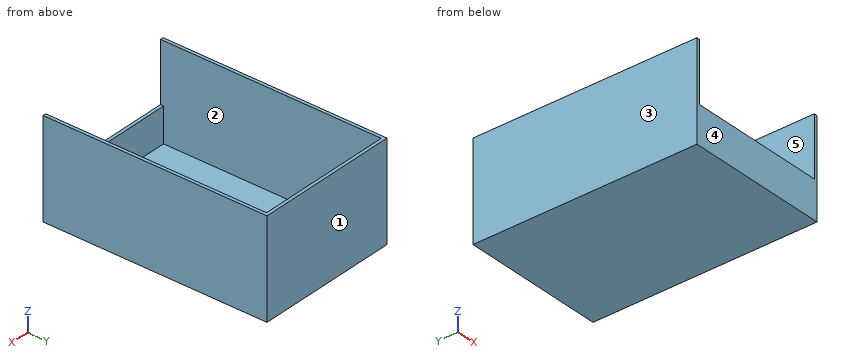
```python
from build123d import *

# Parameters (mm, degrees)
F0_W     = 50.8
F0_H     = 6.35
F0_W_2   = 177.8
F1_DEPTH = 453.39
F2_DEPTH = 6.35
F3_W     = 292.1
F3_H     = 196.85
F4_DEPTH = 6.35


with BuildPart() as f1:
    # F0 (on Front) → F1 (new body)
    with BuildSketch(Plane.XZ):
        Polygon((-139.7, -92.075), (-139.7, -22.225), (-139.7, 98.425), (-146.05, 98.425), (-146.05, -98.425), (-139.7, -98.425), align=None)
        with Locations((-114.3, -95.25)):
            Rectangle(F0_W, F0_H)
        with Locations((114.3, -95.25)):
            Rectangle(F0_W, F0_H)
        Polygon((146.05, -98.425), (146.05, 98.425), (139.7, 98.425), (139.7, -22.225), (139.7, -92.075), (139.7, -98.425), align=None)
        with Locations((0, -95.25)):
            Rectangle(F0_W_2, F0_H)
    extrude(amount=-F1_DEPTH)

    # F0 (on Front) → F2 (join)
    with BuildSketch(Plane.XZ):
        Polygon((139.7, -92.075), (139.7, -22.225), (-139.7, -22.225), (-139.7, -92.075), (-88.9, -92.075), (88.9, -92.075), align=None)
        with Locations((0, -95.25)):
            Rectangle(F0_W_2, F0_H)
        with Locations((-114.3, -95.25)):
            Rectangle(F0_W, F0_H)
        with Locations((114.3, -95.25)):
            Rectangle(F0_W, F0_H)
    extrude(amount=-F2_DEPTH)

    # F3 (on face) → F4 (join)
    with BuildSketch(Plane(origin=(0, 453.39, 0), x_dir=(-1, 0, 0), z_dir=(0, 1, 0))):
        Rectangle(F3_W, F3_H)
    extrude(amount=-F4_DEPTH)


solid = f1.part
```
Geometry check sheet. Reference: the model listing, model coordinates, mm. Face numbers are marked on the shaded views. A direction names the side the tool comes from. Give positions to 0.01 mm unless a question says otherwise; leave off trailing zeros. Order: outer loops, then holes, each group sorted by start corner. A loop starts at its lowest first (then second) coordinate and runs counter-clockwise, first axis right, second up. Notation, with made-up numbers: (31, 72) - (50, 72) arc R33 ccw to (50, 107) - close; hole circle Ø10 at (29.25, 35.5). An arc over 180 degrees is marked (long way). Answer in a Markdown table with one row per item. Add a question column.
Q1. Cross-section at B-B, the plane y = 181.5. Enter the section's corners in (x, z) (3 decimals).
Q2. Cross-section at A-A, the plane z = -76. Enter the section's corners in (x, y), then the cut area to 3 significant figures.
Q3. Tool access check on the marked faces 1 and 2. Record the directions out of +Z, -Z, +X, -X, +Y, -Y that give a thin tool (end or side, any length) a straight path to the whole face; none if there is none.
Q4. Cross-section at C-C, the plane x = 36. Enter the section's corners in (y, z) (3 decimals), then the cut area to 3 significant figures.
Q5. Material ranges on probe 1 along X at (y, z) = (343, -78.5); probe 2 along Y at (x, z) = (-125, -40); probe 3 along Z at (x, y) = (-118, 33.5) (3 decimals), recorded low to high. Write a range as from..to.
Q6. Gauge pin test, flat ends, axial feed: pin 1 (2 mm diameter, centred on x = 115, z = -19, fed in from -Y); pin 2 (8 mm diameter, centred on x = -85, y = 384.5, fed in from +Z) (3 decimals); pin 3 (3 mm diameter, centred on x = -37.5, y = 2.5, fed in from +Z) (3 decimals). Record the tip position at first contact, or that the pin passes through.
Q7. Mould release check, pull along X, two halves, no side actions. Record for the marked faces 3, 4 and 5: pulls with the +X half, pulls with the -X half, needs draft (parallel to the pull), parting line crosses it, or undercut.
Check values:
| question | item | result |
|---|---|---|
| 1 | outline | (-146.05, -98.425) - (146.05, -98.425) - (146.05, 98.425) - (139.7, 98.425) - (139.7, -92.075) - (-139.7, -92.075) - (-139.7, 98.425) - (-146.05, 98.425) - close |
| 2 | outline | (-146.05, 0) - (146.05, 0) - (146.05, 453.39) - (-146.05, 453.39) - close; hole (-139.7, 6.35) - (139.7, 6.35) - (139.7, 447.04) - (-139.7, 447.04) - close |
| 2 | area | 9,310 mm^2 |
| 3 | face 1 | +Z, -Z, +X, -X, +Y |
| 3 | face 2 | +Z |
| 4 | outline | (0, -98.425) - (453.39, -98.425) - (453.39, 98.425) - (447.04, 98.425) - (447.04, -92.075) - (6.35, -92.075) - (6.35, -22.225) - (0, -22.225) - close |
| 4 | area | 4,530 mm^2 |
| 5 | probe 1 | x = -146.05..-139.7, 139.7..146.05 |
| 5 | probe 2 | y = 0..6.35, 447.04..453.39 |
| 5 | probe 3 | z = -98.425..-92.075 |
| 6 | pin 1 | stops at y = 447.04 |
| 6 | pin 2 | stops at z = -92.075 |
| 6 | pin 3 | stops at z = -22.225 |
| 7 | face 3 | pulls with the -X half |
| 7 | face 4 | needs draft |
| 7 | face 5 | undercut |
